The listing builds one solid part. Answer for the finished solid, in the listing's coordinates (mm). A direction names the side the tool comes from. Coordinates: 2 decimals unless noted, no trailing zeros. Write each loop counter-clockwise with the first axis right and the second up, starting at its lowest first coordinate (ties: lowest second). Pieces come first, ordered by that corner, then holes.
from build123d import *

# Parameters (mm, degrees)
EXTRUDE_1_DEPTH     = 3
SKETCH_2_R          = 1
CUT_EXTRUDE_1_DEPTH = 4
SKETCH_3_W          = 20.4
SKETCH_3_H          = 20
CUT_EXTRUDE_2_DEPTH = 4
EXTRUDE_1_2_DEPTH   = 3
FILLET_1_R          = 1
FILLET_2_R          = 1.5


with BuildPart() as part:
    # 草图1 → Extrude 1 (new body)
    with BuildSketch(Plane.XY):
        Polygon((15.2, -15), (-15.2, -15), (-15.2, -6), (-19.2, -6), (-19.2, 6), (-15.2, 6), (-15.2, 15), (15.2, 15), (15.2, 6), (19.2, 6), (19.2, -6), (15.2, -6), align=None)
    extrude(amount=EXTRUDE_1_DEPTH)

    # 草图2 → 切除-拉伸1 (cut, through all)
    with BuildSketch(Plane.XY.offset(3)):
        with Locations((-15.2, 7)):
            Circle(SKETCH_2_R)
        with Locations((-15.2, -7)):
            Circle(SKETCH_2_R)
        with Locations((15.2, -7)):
            Circle(SKETCH_2_R)
        with Locations((15.2, 7)):
            Circle(SKETCH_2_R)
    extrude(amount=-CUT_EXTRUDE_1_DEPTH, mode=Mode.SUBTRACT)

    # 草图3 → 切除-拉伸2 (cut, through all)
    with BuildSketch(Plane.XY.offset(3)):
        Rectangle(SKETCH_3_W, SKETCH_3_H)
    extrude(amount=-CUT_EXTRUDE_2_DEPTH, mode=Mode.SUBTRACT)

    # 草图4 → Extrude 1 2 (add)
    with BuildSketch(Plane.XY.offset(3)):
        Polygon((-11.600142822, 8.571854322), (8.799857178, -11.428145678), (11.600142822, -8.571854322), (-8.799857178, 11.428145678), align=None)
        Polygon((-8.799857178, -11.428145678), (11.600142822, 8.571854322), (8.799857178, 11.428145678), (-11.600142822, -8.571854322), align=None)
    extrude(amount=-EXTRUDE_1_2_DEPTH)

    # 圆角1
    fillet_1_edges = [part.edges().sort_by_distance(p)[0] for p in [
        (-15.2, 15, 1.5),
        (15.2, 15, 1.5),
        (19.2, 6, 1.5),
        (19.2, -6, 1.5),
        (15.2, -15, 1.5),
        (-15.2, -15, 1.5),
        (-19.2, -6, 1.5),
        (-19.2, 6, 1.5),
    ]]
    fillet(fillet_1_edges, radius=FILLET_1_R)

    # 圆角2
    fillet_2_edges = [part.edges().sort_by_distance(p)[0] for p in [
        (-2.856851414, 0, 1.5),
        (0, 2.800834719, 1.5),
        (2.856851414, 0, 1.5),
        (0, -2.800834719, 1.5),
        (-7.343148586, -10, 1.5),
        (7.343148586, -10, 1.5),
        (10.2, 7.199165281, 1.5),
        (10.2, -7.199165281, 1.5),
        (7.343148586, 10, 1.5),
        (-7.343148586, 10, 1.5),
        (-10.2, -7.199165281, 1.5),
        (-10.2, 7.199165281, 1.5),
    ]]
    fillet(fillet_2_edges, radius=FILLET_2_R)


solid = part.part
Q1. Find the intervals of material crossed by probe 1 along X at (y, z) = (4.75, 2.75); probe 2 along X at (y, z) = (-2.25, 0.75); probe 3 along Y at (x, z) = (-0.5, 1.55), in increasing order.
Answers below:
probe 1: x = -19.2 to -9.7, -7.7 to -1.99, 1.99 to 7.7, 9.7 to 19.2
probe 2: x = -19.2 to -10.2, -5.15 to 5.15, 10.2 to 19.2
probe 3: y = -15 to -10, -3.49 to 3.49, 10 to 15
Q2. The part is cut by section B-B, the plane y = 9.25. Write down the section's boundary in (x, z).
Answers below:
outline: (-15.2, 0) - (-4.97, 0) - (-4.97, 3) - (-15.2, 3) - close; (4.97, 0) - (15.2, 0) - (15.2, 3) - (4.97, 3) - close
Q3. The part is cut by section D-D, the plane z = 1.85. State how many separate pieces and enclosed holes the cut face has, then the cut area to 3 significant figures.
Answers below:
separate pieces: 1
enclosed holes: 4
area: 813 mm2
Q4. The part is cut by section A-A, the plane x = -1.5. Write down the section's boundary in (y, z), then the cut area to 3 significant figures.
Answers below:
outline: (-15, 0) - (-10, 0) - (-10, 3) - (-15, 3) - close; (-4.27, 0) - (4.27, 0) - (4.27, 3) - (-4.27, 3) - close; (10, 0) - (15, 0) - (15, 3) - (10, 3) - close
area: 55.6 mm2
Q5. Given pin 1 (0.9 mm diameter, centred on y = 10.5, z = 1, fed in from +X), flat-ended and moving along its own axis, determine where the tip first touches the part or whether it passes through.
Answers below:
pin 1: stops at x = 15.2
Q6. Determine the mould class of faces 1 (the face through (18.915, 5.699, 1.521)), 2 (the face through (9.304, 5.001, 1.479)), 3 (the face through (0, 0, 0)) for opening direction Y: released by +Y, released by -Y, zero draft, split by the parting line, or undercut.
Answers below:
face 1: released by +Y
face 2: undercut
face 3: zero draft
Q7. The part is cut by section C-C, the plane y = -1.75. Write down the section's boundary in (x, z).
Answers below:
outline: (-19.2, 0) - (-10.2, 0) - (-10.2, 3) - (-19.2, 3) - close; (-4.64, 0) - (4.64, 0) - (4.64, 3) - (-4.64, 3) - close; (10.2, 0) - (19.2, 0) - (19.2, 3) - (10.2, 3) - close
Q8. Which of the six approach directions +Z, -Z, +X, -X, +Y, -Y give full straight-line access (tool end or side, diameter ignored) to faces 4 (the face through (0, 0, 3)), 5 (the face through (0, -10, 2)), 6 (the face through (0, -15, 1)), 7 (the face through (17, 6, 1)), 8 (the face through (-17, 6, 1))?
Answers below:
face 4: +Z, +X, -X, +Y, -Y
face 5: +Z, -Z
face 6: +Z, -Z, +X, -X, -Y
face 7: +Z, -Z, +X, +Y
face 8: +Z, -Z, -X, +Y
